Input: part model. Units: mm. Frame: model coordinates. A direction names the side the tool comes from. Round coordinates to 2 decimals unless told otherwise and drop trailing zeros. Order: outer loops, then holes, each group sorted by start corner. A loop starts at its lowest first (then second) coordinate and runs counter-clockwise, first axis right, second up. Notation, with made-up numbers: (22, 72.5) -> (74, 72.5) arc R24 ccw to (74, 95.5) -> close; hole circle Ø9 at (-4, -6). An arc over 180 degrees is marked (long way). Use a Markdown table: item, result.
from build123d import *

# Parameters (mm, degrees)
SKETCH1_R           = 4
BOSS_EXTRUDE1_DEPTH = 15
BOSS_EXTRUDE2_DEPTH = 5


with BuildPart() as part:
    # Sketch1 → Boss-Extrude1 (new body)
    with BuildSketch(Plane(origin=(0, 0, 0), x_dir=(1, 0, 0), z_dir=(0, 1, 0))):
        with Locations(Location((0, 0, 0), (0, 0, 270))):
            Circle(SKETCH1_R)
    extrude(amount=BOSS_EXTRUDE1_DEPTH)

    # Sketch2 → Boss-Extrude2 (add)
    with BuildSketch(Plane(origin=(0, 15, 0), x_dir=(1, 0, 0), z_dir=(0, 1, 0))):
        Polygon((0, -8.082903769), (7, -4.041451884), (7, 4.041451884), (0, 8.082903769), (-7, 4.041451884), (-7, -4.041451884), align=None)
    extrude(amount=BOSS_EXTRUDE2_DEPTH)

    # Sketch4 → Cut-Revolve2 (revolve, cut)
    with BuildSketch(Plane(origin=(0, 0, 0), x_dir=(0, 0, -1), z_dir=(1, 0, 0)), mode=Mode.PRIVATE) as cut_revolve2_sk:
        with BuildLine():
            Line((-6.082903769, 20), (-8.082903769, 20))
            Line((-8.082903769, 20), (-8.082903769, 18))
            ThreePointArc((-8.082903769, 18), (-7.497117331, 19.414213562), (-6.082903769, 20))
        make_face()
    revolve(cut_revolve2_sk.sketch.rotate(Axis((0, 0, 0), (0, 1, 0)), 180), axis=Axis((0, 0, 0), (0, 1, 0)), mode=Mode.SUBTRACT)


solid = part.part
1) Ray query, probe 1 along Y at (x, z) = (5.25, -2.25); probe 2 along X at (y, z) = (9.5, 0); probe 3 along Z at (x, y) = (1.5, 19). Return the intervals inside material, ascending.
Answer key:
| item | result |
|---|---|
| probe 1 | y = 15 to 20 |
| probe 2 | x = -4 to 4 |
| probe 3 | z = -7.22 to 7.22 |
2) Cut plane A-A on z = 0. Return loops of the section in (x, y).
Answer key:
| item | result |
|---|---|
| outline | (-7, 15) -> (-4, 15) -> (-4, 0) -> (4, 0) -> (4, 15) -> (7, 15) -> (7, 19.78) arc R2 ccw to (6.08, 20) -> (-6.08, 20) arc R2 ccw to (-7, 19.78) -> close |
3) Set-up query: faces 1 (the face through (-7, 17, 0)), 2 (the face through (-3.905, 7.395, -0.867)). Return all of +Z, -Z, +X, -X, +Y, -Y with unobstructed straight access to the full face (end or side cutting, diameter ignored); none if empty.
Answer key:
| item | result |
|---|---|
| face 1 | +Z, -Z, -X, +Y, -Y |
| face 2 | -Y |
4) Contact query for flat-ended pins moving along their axis: P1, Ø2, axis at x = -4, y = 11, coming from the -Z side; P2, Ø1.5, axis at x = -2.5, y = 11, coming from the -Z side; P3, Ø3, axis at x = -2, y = 6.5, coming from the +Z side. Output: stop coordinate, or through.
Answer key:
| item | result |
|---|---|
| P1 | stops at z = -2.65 |
| P2 | stops at z = -3.6 |
| P3 | stops at z = 3.97 |
5) Cut plane B-B on y = 18.75. Return loops of the section in (x, z).
Answer key:
| item | result |
|---|---|
| outline | (-7, -3.74) arc R7.94 ccw to (-6.74, -4.19) -> (-0.26, -7.93) arc R7.94 ccw to (0.26, -7.93) -> (6.74, -4.19) arc R7.94 ccw to (7, -3.74) -> (7, 3.74) arc R7.94 ccw to (6.74, 4.19) -> (0.26, 7.93) arc R7.94 ccw to (-0.26, 7.93) -> (-6.74, 4.19) arc R7.94 ccw to (-7, 3.74) -> close |
6) Cut plane C-C on y = 14.5. Return loops of the section in (x, z), and give its area (3 significant figures).
Answer key:
| item | result |
|---|---|
| outline | circle Ø8 at (0, 0) |
| area | 50.3 mm^2 |
